Design review of the part built by this model. Coordinates are the model's own, in mm. Give positions to 0.01 mm unless a question says otherwise; leave off trailing zeros. Write each loop counter-clockwise with the first axis right and the second up, starting at its lowest first coordinate (ties: lowest second). Pieces come first, ordered by that corner, then holes. Notation, with made-up numbers: (3, 16) - (46, 16) arc R9 cw to (46, 31) - close; hole circle Ø4 at (-40, 65.5). An arc over 180 degrees is marked (long way). Use a Markdown table: item, result. Add a question column.
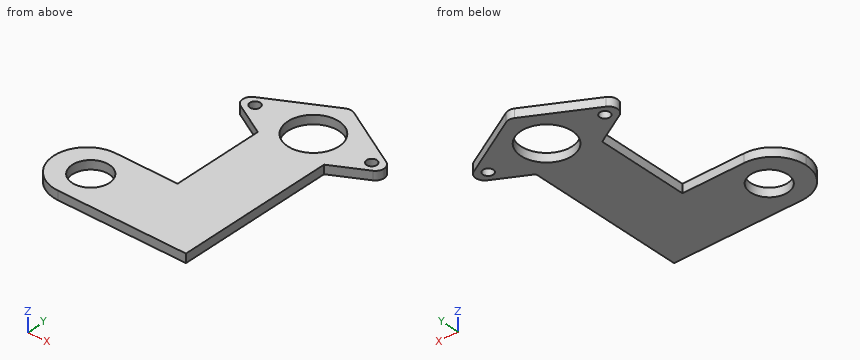
```python
from build123d import *

# Parameters (mm, degrees)
SKETCH1_R           = 3.5
SKETCH1_R_2         = 17.5
SKETCH1_R_3         = 12.7
BOSS_EXTRUDE1_DEPTH = 6


with BuildPart() as part:
    # Sketch1 → Boss-Extrude1 (new body)
    with BuildSketch(Plane.XY):
        with BuildLine():
            Line((-45.343148698, -5.267373437), (-22.7, -17.618181818))
            Line((-22.7, -17.618181818), (-22.7, -80.51))
            Line((-22.7, -80.51), (-65.01, -80.51))
            ThreePointArc((-65.01, -80.51), (-81.054252865, -87.155747135), (-87.7, -103.2))
            Line((-87.7, -103.2), (-87.7, -103.22))
            ThreePointArc((-87.7, -103.22), (-81.054252865, -119.264252865), (-65.01, -125.91))
            Line((-65.01, -125.91), (22.7, -125.91))
            Line((22.7, -125.91), (22.7, -17.618181818))
            Line((22.7, -17.618181818), (45.343148698, -5.267373437))
            ThreePointArc((45.343148698, -5.267373437), (47.629429129, -3.062786582), (48.470035914, 0))
            ThreePointArc((48.470035914, 0), (47.629429129, 3.062786582), (45.343148698, 5.267373437))
            Line((45.343148698, 5.267373437), (2.873112784, 28.432847572))
            ThreePointArc((2.873112784, 28.432847572), (0, 29.165474135), (-2.873112784, 28.432847572))
            Line((-2.873112784, 28.432847572), (-45.343148698, 5.267373437))
            ThreePointArc((-45.343148698, 5.267373437), (-48.470035914, 0), (-45.343148698, -5.267373437))
        make_face()
        with Locations((-40, 0)):
            Circle(SKETCH1_R, mode=Mode.SUBTRACT)
        Circle(SKETCH1_R_2, mode=Mode.SUBTRACT)
        with Locations((40, 0)):
            Circle(SKETCH1_R, mode=Mode.SUBTRACT)
        with Locations((-62.35, -103.21)):
            Circle(SKETCH1_R_3, mode=Mode.SUBTRACT)
    extrude(amount=BOSS_EXTRUDE1_DEPTH)


solid = part.part
```
(1) For line 1 along Y through (x, z) = (-40, 1.7); line 2 along Y through (x, z) = (0, 1.6); line 3 along X through (y, z) = (-3, 3.8), list the stretches that pass through material, from the lowest coordinate up.
(2) Add section B-B (y = 12). State the section outline as (x, z) points.
(3) Insertion check: pin 1 (3 mm diameter, centred on y = -36.5, z = 3.5, fed in from -X); pin 2 (1 mm diameter, centred on x = -74, z = 1, fed in from -Y); pin 3 (1.8 mm diameter, centred on y = -86, z = 3, fed in from +X). Each pin has a flat end and moves straight along its axis. Give the tip position at first contact, or say it passes through.
(4) Add section D-D (x = -40). State the section outline as (y, z) points, and give its area (3 significant figures).
(5) Add section A-A (x = 0). State the section outline as (y, z) points.
(6) Add section C-C (z = 2.2). Count the separate pieces of the cut face and the enclosed holes in it, and give its area (3 significant figures).
Answers follow:
| question | item | result |
|---|---|---|
| 1 | line 1 | -125.91 to -80.51, -8.18 to -3.5, 3.5 to 8.18 |
| 1 | line 2 | -125.91 to -17.5, 17.5 to 29.17 |
| 1 | line 3 | -47.67 to -41.8, -38.2 to -17.24, 17.24 to 38.2, 41.8 to 47.67 |
| 2 | outline | (-33, 0) - (-12.74, 0) - (-12.74, 6) - (-33, 6) - close; (12.74, 0) - (33, 0) - (33, 6) - (12.74, 6) - close |
| 3 | pin 1 | x = -22.7 |
| 3 | pin 2 | y = -124.26 |
| 3 | pin 3 | x = 22.7 |
| 4 | outline | (-125.91, 0) - (-80.51, 0) - (-80.51, 6) - (-125.91, 6) - close; (-8.18, 0) - (-3.5, 0) - (-3.5, 6) - (-8.18, 6) - close; (3.5, 0) - (8.18, 0) - (8.18, 6) - (3.5, 6) - close |
| 4 | area | 329 mm^2 |
| 5 | outline | (-125.91, 0) - (-17.5, 0) - (-17.5, 6) - (-125.91, 6) - close; (17.5, 0) - (29.17, 0) - (29.17, 6) - (17.5, 6) - close |
| 6 | separate pieces | 1 |
| 6 | enclosed holes | 4 |
| 6 | area | 9,060 mm^2 |
